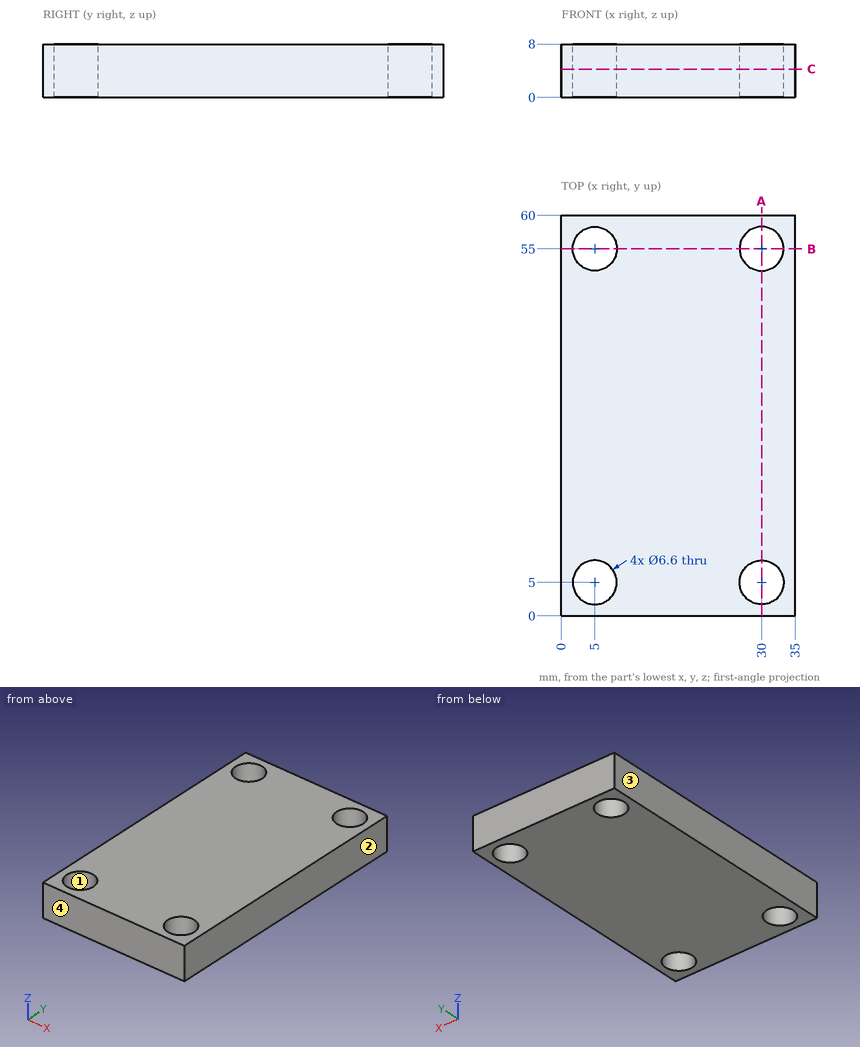
Design review of the part shown in the three views and the two pictorial views. Dimensions are in mm from the part's minimum x, y and z. Round coordinates to 2 decimals unless told otherwise and drop trailing zeros. Write each loop counter-clockwise with the first axis right and the second up, starting at its lowest first coordinate (ties: lowest second). Pieces come first, ordered by that corner, then holes.
Item 1: Wall thickness on L1, parallel to X at y = 55, z = 3.25; L2, parallel to Y at x = 5, z = 4.5: over which ranges is each line inside the solid? List them lowest first.
Item 2: For pin 1 Ø10.5 at (x, y) = (30, 55) entering from +Z, flat-tipped, find the tip position at first contact; note if it passes through.
Item 3: Consider section B-B on y = 55. Give the boundary of the cut face in (x, z).
Item 4: Consider section A-A on x = 30. Give the boundary of the cut face in (y, z), and give its area (3 significant figures).
Item 5: Draft analysis for pull direction X (two halves, no side actions). For the marked faces 1, 2, 3 and 4, state which applies: released by +X, released by -X, zero draft, split by the parting line, or undercut.
Item 6: Consider section C-C on z = 4.25. Give the boundary of the cut face in (x, y).
Check values:
1. L1: x = 0 to 1.7, 8.3 to 26.7, 33.3 to 35
1. L2: y = 0 to 1.7, 8.3 to 51.7, 58.3 to 60
2. pin 1: stops at z = 8
3. outline: (0, 0) - (1.7, 0) - (1.7, 8) - (0, 8) - close; (8.3, 0) - (26.7, 0) - (26.7, 8) - (8.3, 8) - close; (33.3, 0) - (35, 0) - (35, 8) - (33.3, 8) - close
4. outline: (0, 0) - (1.7, 0) - (1.7, 8) - (0, 8) - close; (8.3, 0) - (51.7, 0) - (51.7, 8) - (8.3, 8) - close; (58.3, 0) - (60, 0) - (60, 8) - (58.3, 8) - close
4. area: 374 mm2
5. face 1: undercut
5. face 2: released by +X
5. face 3: released by -X
5. face 4: zero draft
6. outline: (0, 0) - (35, 0) - (35, 60) - (0, 60) - close; hole circle Ø6.6 at (5, 5); hole circle Ø6.6 at (5, 55); hole circle Ø6.6 at (30, 5); hole circle Ø6.6 at (30, 55)
